Design review of the part built by this model. Coordinates are the model's own, in mm. A direction names the side the tool comes from. Give positions to 0.01 mm unless a question says otherwise; leave off trailing zeros. Loops run counter-clockwise (first coordinate to the right, second up) from the corner with the lowest first, then second, coordinate; pieces in that order, holes last. Notation, with made-up numbers: M -7,-2 L 20,-2 A14 cw 20,19 Z; hole C 85,47.25 d5. An arc over 180 degrees is marked long. Use CSV: the item, a comma, the result in double quotes.
Autodesk Inventor part; units mm, degrees
ref_plane "YZ Plane" through (0, 0, 0) normal (1, 0, 0) x (0, 1, 0)
ref_plane "XZ Plane" through (0, 0, 0) normal (0, 1, 0) x (-1, 0, 0)
ref_plane "XY Plane" through (0, 0, 0) normal (0, 0, 1) x (1, 0, 0)
sketch "Sketch1" plane through (0, 0, 0) normal (0, 0, 1) x (1, 0, 0)
  line L0 (-67.183, -7.8688) -> (-67.183, 109.1349)
  line L1 (-67.183, -7.8688) -> (-60.833, -7.8688)
  line L2 (-67.183, 109.1349) -> (-95.25, 109.1349)
  line L3 (-95.25, 109.1349) -> (-95.25, 121.8349)
  line L4 (-95.25, 121.8349) -> (-88.9, 121.8349)
  line L5 (-88.9, 121.8349) -> (-88.9, 147.2349)
  line L6 (-88.9, 147.2349) -> (-38.3236, 147.2349) construction
  line L7 (-60.833, -7.8688) -> (-33.1797, 95.3346)
  line L8 (-33.1797, 95.3346) -> (-53.4136, 95.3346)
  line L9 (0, -38.8896) -> (0, 178.2557)
  line L10 (-88.9, 147.2349) -> (-48.411, 128.3546)
  line L11 (-48.411, 128.3546) -> (-53.4136, 128.3546)
  line L12 (-53.4136, 128.3546) -> (-53.4136, 95.3346)
  point P0 (0, 0)
  dimension "d0" = 6.35
  dimension "d1" = 60.833
  dimension "d4" = 12.7
  dimension "d5" = 28.067
  dimension "d6" = 25.4
  dimension "d9" = 6.35
  dimension "d10" = 105
  dimension "d16" = 20.2339
  dimension "d17" = 25
  dimension "d18" = 5.0026
  dimension "d19" = 33.02
  dimension "d20" = 33.1797
  dimension "d21" = 95.25
  dimension "d22" = 117.0038
revolve "Revolution1" add sketch "Sketch1" angle 360 about axis through (0, -10, 0) along (0, 1, 0)
properties part number "Phenlic"
(1) The part is to be moulded in two halves that separate along X. For faces 4 (the flat face through (35, -7.869, 50)), 5 (the cylindrical face through (75.587, 115.574, -57.958)), 6 (the cylindrical face through (42, 112, 33)), say which applies: released by +X, released by -X, zero draft, split by the parting line, or undercut.
A:
face 4,"zero draft"
face 5,"split by the parting line"
face 6,"undercut"
(2) We need section D-D on y = 14. State the section outline as (x, z) points.
A:
outline,"C 0,0 d134.37; hole C 0,0 d109.95"
(3) We need section C-C on y = 90.5. State the section outline as (x, z) points, then the cut area to 3 significant figures.
A:
outline,"C 0,0 d134.37; hole C 0,0 d68.95"
area,"10,400 mm²"
(4) We need section A-A on x = 0. State the section outline as (y, z) points, then the cut area to 3 significant figures.
A:
outline,"M -7.87,-67.18 L 109.13,-67.18 L 109.13,-95.25 L 121.83,-95.25 L 121.83,-88.9 L 147.23,-88.9 L 128.35,-48.41 L 128.35,-53.41 L 95.33,-53.41 L 95.33,-33.18 L -7.87,-60.83 Z; M -7.87,60.83 L 95.33,33.18 L 95.33,53.41 L 128.35,53.41 L 128.35,48.41 L 147.23,88.9 L 121.83,88.9 L 121.83,95.25 L 109.13,95.25 L 109.13,67.18 L -7.87,67.18 Z"
area,"6,830 mm²"
(5) Wall thickness on line 1 along Z through (x, y) = (0, 105.5); line 2 along Z through (x, y) = (0, 121); line 3 along X through (y, z) = (3.5, -47): over which ranges is each line inside the solid? List them lowest first. Write a range as [from, to].
A:
line 1,"[-67.18, -53.41], [53.41, 67.18]"
line 2,"[-95.25, -53.41], [53.41, 95.25]"
line 3,"[-48.01, -33.62], [33.62, 48.01]"
(6) We need section B-B on z = 0. State the section outline as (x, y) points, then the cut area to 3 significant figures.
A:
outline,"M -95.25,109.13 L -67.18,109.13 L -67.18,-7.87 L -60.83,-7.87 L -33.18,95.33 L -53.41,95.33 L -53.41,128.35 L -48.41,128.35 L -88.9,147.23 L -88.9,121.83 L -95.25,121.83 Z; M 33.18,95.33 L 60.83,-7.87 L 67.18,-7.87 L 67.18,109.13 L 95.25,109.13 L 95.25,121.83 L 88.9,121.83 L 88.9,147.23 L 48.41,128.35 L 53.41,128.35 L 53.41,95.33 Z"
area,"6,830 mm²"
(7) Machinability: for faces 1 (the flat face through (28, 128.355, 40)), 2 (the flat face through (78, 121.835, 43)), 3 (the cylindrical face through (14.564, 51.452, -65.585)), which of the approach directions +Z, -Z, +X, -X, +Y, -Y give a long, thin tool a straight path to every point of the face, cutting with its end or side? Answer none if there is none.
A:
face 1,"none"
face 2,"+Y"
face 3,"-Y"
(8) Clearance check with flat-ended pins moving along their axes: P1, Ø2, axis at x = -30.5, y = 40, coming from the +Z side; P2, Ø10, axis at y = 57, z = -3.5, coming from the +X side; P3, Ø12, axis at y = 124.5, z = -58, coming from the +X side. State where each tip first meets the part, or that it passes through.
A:
P1,"z = 60.36"
P2,"x = 67.18"
P3,"x = 79.39"
